from build123d import *

# Parameters (mm, degrees)
BOSS_EXTRUDE1_DEPTH = 0.87376
SKETCH2_R           = 9.398
CUT_EXTRUDE1_DEPTH  = 0.87376


with BuildPart() as part:
    # Sketch1 → Boss-Extrude1 (new body)
    with BuildSketch(Plane.YZ):
        with BuildLine():
            Line((0, 0), (0, 76.2))
            ThreePointArc((0, 76.2), (12.7, 88.9), (25.4, 76.2))
            Line((25.4, 76.2), (25.4, 0))
            ThreePointArc((25.4, 0), (12.7, -12.7), (0, 0))
        make_face()
    extrude(amount=BOSS_EXTRUDE1_DEPTH)

    # Sketch2 → Cut-Extrude1 (cut)
    with BuildSketch(Plane.YZ):
        with Locations(Location((12.7, 76.2, 0), (0, 0, 90))):
            Circle(SKETCH2_R)
        with Locations(Location((12.7, 0, 0), (0, 0, 90))):
            Circle(SKETCH2_R)
    extrude(amount=CUT_EXTRUDE1_DEPTH, mode=Mode.SUBTRACT)


solid = part.part
Part model, mm, in its own coordinate system. Give positions to 0.01 mm unless a question says otherwise; leave off trailing zeros. Write each loop counter-clockwise with the first axis right and the second up, starting at its lowest first coordinate (ties: lowest second). Pieces come first, ordered by that corner, then holes.
1) Cut at B-B on x = 0.6. Write the cut outline in (y, z).
Resolved:
outline: (0, 0) arc R12.7 ccw to (25.4, 0) - (25.4, 76.2) arc R12.7 ccw to (0, 76.2) - close; hole circle Ø18.8 at (12.7, 0); hole circle Ø18.8 at (12.7, 76.2)
2) Pin check, flat tip, straight feed: pin 1 (6 mm diameter, centred on y = 21.5, z = 76.5, fed in from -X). Stop position of the tip, or through.
Resolved:
pin 1: stops at x = 0
3) Cut at C-C on z = 78.5. Write the cut outline in (x, y), then the cut area to 3 significant figures.
Resolved:
outline: (0, 0.21) - (0.87, 0.21) - (0.87, 3.59) - (0, 3.59) - close; (0, 21.81) - (0.87, 21.81) - (0.87, 25.19) - (0, 25.19) - close
area: 5.90 mm2
4) Probe L1, parallel to Y at x = 0.7, z = 76.2; L2, parallel to Z at x = 0.55, y = 14.25; L3, parallel to Z at x = 0.7, y = 5.25. List the from-to ranges inside material, lowest first.
Resolved:
L1: y = 0 to 3.3, 22.1 to 25.4
L2: z = -12.61 to -9.27, 9.27 to 66.93, 85.47 to 88.81
L3: z = -10.29 to -5.73, 5.73 to 70.47, 81.93 to 86.49
5) Cut at A-A on y = 17. Write the cut outline in (x, z).
Resolved:
outline: (0, -11.95) - (0.87, -11.95) - (0.87, -8.36) - (0, -8.36) - close; (0, 8.36) - (0.87, 8.36) - (0.87, 67.84) - (0, 67.84) - close; (0, 84.56) - (0.87, 84.56) - (0.87, 88.15) - (0, 88.15) - close
6) Two-plate mould, pull along X, no slides. Class faces 1 (the face through (0.431, 12.979, -12.697)), 2 (the face through (0.874, 13, 39)), 3 (the face through (0, 13, 39)): released by +X, released by -X, zero draft, split by the parting line, or undercut.
Resolved:
face 1: zero draft
face 2: released by +X
face 3: released by -X
7) Cut at D-D on y = 12.7. Write the cut outline in (x, z).
Resolved:
outline: (0, -12.7) - (0.87, -12.7) - (0.87, -9.4) - (0, -9.4) - close; (0, 9.4) - (0.87, 9.4) - (0.87, 66.8) - (0, 66.8) - close; (0, 85.6) - (0.87, 85.6) - (0.87, 88.9) - (0, 88.9) - close
